```python
from build123d import *

# Parameters (mm, degrees)
SKETCH1_W           = 190.5
SKETCH1_H           = 95.25
BOSS_EXTRUDE1_DEPTH = 6.35
SKETCH2_R           = 3.96875
CUT_EXTRUDE1_DEPTH  = 7.35
SKETCH3_W           = 6.35
SKETCH3_H           = 12.7
CUT_EXTRUDE2_DEPTH  = 7.35
SKETCH4_W           = 6.35
SKETCH4_H           = 12.7
CUT_EXTRUDE3_DEPTH  = 7.35
LPATTERN1_COUNT     = 4
LPATTERN1_PITCH     = 25.4
CUT_EXTRUDE4_DEPTH  = 7.35


with BuildPart() as part:
    # Sketch1 → Boss-Extrude1 (new body)
    with BuildSketch(Plane.XY):
        with Locations((95.25, 47.625)):
            Rectangle(SKETCH1_W, SKETCH1_H)
    extrude(amount=BOSS_EXTRUDE1_DEPTH)

    # Sketch2 → Cut-Extrude1 (cut, through all)
    with BuildSketch(Plane.XY.offset(6.35)):
        with Locations((63.5, 38.1)):
            Circle(SKETCH2_R)
    extrude(amount=-CUT_EXTRUDE1_DEPTH, mode=Mode.SUBTRACT)

    # Sketch3 → Cut-Extrude2 (cut, through all)
    with BuildSketch(Plane.XY.offset(6.35)):
        with Locations((3.175, 19.05)):
            Rectangle(SKETCH3_W, SKETCH3_H)
    cut_extrude2 = extrude(amount=-CUT_EXTRUDE2_DEPTH, mode=Mode.SUBTRACT)

    # Sketch4 → Cut-Extrude3 (cut, through all)
    with BuildSketch(Plane.XY.offset(6.35)):
        with Locations((187.325, 19.05)):
            Rectangle(SKETCH4_W, SKETCH4_H)
    cut_extrude3 = extrude(amount=-CUT_EXTRUDE3_DEPTH, mode=Mode.SUBTRACT)

    # LPattern1: Cut-Extrude2, Cut-Extrude3 ×4
    with Locations(*[(0, i * LPATTERN1_PITCH, 0) for i in range(1, LPATTERN1_COUNT)]):
        add(cut_extrude2, mode=Mode.SUBTRACT)
        add(cut_extrude3, mode=Mode.SUBTRACT)

    # Sketch6 → Cut-Extrude4 (cut, through all)
    with BuildSketch(Plane.XY.offset(6.35)):
        Polygon((25.4, 95.25), (25.4, 82.094090512), (123.597045256, 25.4), (165.1, 25.4), (165.1, 95.25), align=None)
        Polygon((25.4, 38.1), (25.4, 25.4), (47.397045256, 25.4), align=None)
    extrude(amount=-CUT_EXTRUDE4_DEPTH, mode=Mode.SUBTRACT)


solid = part.part
```
Check sheet for the modelled part. Datum: model origin and axes. Units: mm. A direction names the side the tool comes from. Give positions to 0.01 mm unless a question says otherwise; leave off trailing zeros. Write each loop counter-clockwise with the first axis right and the second up, starting at its lowest first coordinate (ties: lowest second). Pieces come first, ordered by that corner, then holes.
Item 1: Cross-section at C-C (y = 68). Enter the section's corners in (x, z), and give its area (3 significant figures).
Item 2: Cross-section at A-A (y = 32). Enter the section's corners in (x, z), and give its area (3 significant figures).
Item 3: Draft check along Y on faces 4 (the face through (0, 6, 3)), 5 (the face through (16, 95.25, 3)), 6 (the face through (36.553, 31.661, 3.219)), 7 (the face through (187, 25.4, 3)). Enter one of: released by +Y, released by -Y, zero draft, split by the parting line, or undercut.
Item 4: Access from +Z, -Z, +X, -X, +Y, -Y to the whole of each face (thin tool, end or side, straight path). Record for faces 1 (the face through (6.35, 70, 3)), 2 (the face through (0, 82, 3)), 3 (the face through (187, 38.1, 3)).
Item 5: Gauge pin test, flat ends, axial feed: pin 1 (3 mm diameter, centred on x = 187, z = 2.5, fed in from +Y); pin 2 (3 mm diameter, centred on y = 43.5, z = 4, fed in from -X). Record the tip position at first contact, or that the pin passes through.
Item 6: Cross-section at B-B (x = 63.5). Enter the section's corners in (y, z), and give its area (3 significant figures).
Item 7: Cross-section at D-D (z = 1). Count the separate pieces of the cut face and the enclosed holes in it, and give its area (3 significant figures).
Item 8: Scan lines: L1, parallel to X at y = 91.5, z = 0.5; L2, parallel to Y at x = 137.5, z = 2; L3, parallel to X at y = 20.5, z = 4. Record each from-to range of solid material in increasing order.
Report:
1. outline: (6.35, 0) - (49.81, 0) - (49.81, 6.35) - (6.35, 6.35) - close; (165.1, 0) - (184.15, 0) - (184.15, 6.35) - (165.1, 6.35) - close
1. area: 397 mm2
2. outline: (0, 0) - (25.4, 0) - (25.4, 6.35) - (0, 6.35) - close; (35.97, 0) - (112.17, 0) - (112.17, 6.35) - (35.97, 6.35) - close; (165.1, 0) - (190.5, 0) - (190.5, 6.35) - (165.1, 6.35) - close
2. area: 806 mm2
3. face 4: zero draft
3. face 5: released by +Y
3. face 6: undercut
3. face 7: undercut
4. face 1: +Z, -Z, -X
4. face 2: +Z, -Z, -X, +Y, -Y
4. face 3: +Z, -Z, +X
5. pin 1: stops at y = 88.9
5. pin 2: stops at x = 6.35
6. outline: (0, 0) - (34.13, 0) - (34.13, 6.35) - (0, 6.35) - close; (42.07, 0) - (60.1, 0) - (60.1, 6.35) - (42.07, 6.35) - close
6. area: 331 mm2
7. separate pieces: 1
7. enclosed holes: 2
7. area: 10,400 mm2
8. L1: x = 6.35 to 25.4, 165.1 to 184.15
8. L2: y = 0 to 25.4
8. L3: x = 6.35 to 184.15
